from build123d import *

# Parameters (mm, degrees)
PAD_DEPTH            = 14
SKETCH001_R          = 12.7
POCKET_DEPTH         = 10
SKETCH002_R          = 3.2
POCKET001_DEPTH      = 20.001
POCKET001_DEPTH_BACK = -20.001
CHAMFER_SIZE         = 0.6


with BuildPart() as part:
    # Sketch → Pad (new body)
    with BuildSketch(Plane.XY):
        with BuildLine():
            Line((-36.717816, 3.612355), (-4.294539, 19.030888))
            ThreePointArc((4.294539, 19.030888), (0, 20), (-4.294539, 19.030888))
            Line((4.294539, 19.030888), (36.717816, 3.612355))
            ThreePointArc((36.717816, -3.612355), (39, 0), (36.717816, 3.612355))
            Line((36.717816, -3.612355), (4.294539, -19.030888))
            ThreePointArc((-4.294539, -19.030888), (0, -20), (4.294539, -19.030888))
            Line((-4.294539, -19.030888), (-36.717816, -3.612355))
            ThreePointArc((-36.717816, 3.612355), (-39, 0), (-36.717816, -3.612355))
        make_face()
    extrude(amount=PAD_DEPTH)

    # Sketch001 → Pocket (cut)
    with BuildSketch(Plane.XY):
        Circle(SKETCH001_R)
    extrude(amount=POCKET_DEPTH, mode=Mode.SUBTRACT)

    # Sketch002 → Pocket001 (cut, two sides)
    with BuildSketch(Plane(origin=(0, 0, -1), x_dir=(1, 0, 0), z_dir=(0, -1, 0))) as pocket001_sk:
        with Locations((0, 7)):
            Circle(SKETCH002_R)
    extrude(amount=-POCKET001_DEPTH, mode=Mode.SUBTRACT)
    extrude(pocket001_sk.sketch, amount=-POCKET001_DEPTH_BACK, mode=Mode.SUBTRACT)

    # Chamfer
    chamfer_edges = [part.edges().sort_by_distance(p)[0] for p in [
        (-20.506178, 11.321621, 0),
        (-39, 0, 0),
        (0, 20, 0),
        (-20.506178, -11.321621, 0),
        (20.506178, 11.321621, 0),
        (0, -20, 0),
        (39, 0, 0),
        (20.506178, -11.321621, 0),
        (-12.7, 0, 0),
        (-20.506178, 11.321621, 14),
        (0, 20, 14),
        (20.506178, 11.321621, 14),
        (39, 0, 14),
        (20.506178, -11.321621, 14),
        (0, -20, 14),
        (-20.506178, -11.321621, 14),
        (-39, 0, 14),
        (-3.2, -19.474175, 6),
        (-3.2, 19.474175, 6),
    ]]
    chamfer(chamfer_edges, length=CHAMFER_SIZE)


solid = part.part
Design review of the part built by this model. Coordinates are the model's own, in mm. A direction names the side the tool comes from. Coordinates: 2 decimals unless noted, no trailing zeros. Order: outer loops, then holes, each group sorted by start corner. A loop starts at its lowest first (then second) coordinate and runs counter-clockwise, first axis right, second up.
Item 1: Take a section at D-D, the plane x = 0. Count the separate pieces of the cut face and the enclosed holes in it, then the cut area to 3 significant figures.
Item 2: For faces 1 (the flat face through (0, 0, 10)), 2 (the cylindrical face through (39, 0, 7)), list the 3-axis set-ups (+Z, -Z, +X, -X, +Y, -Y) from which the entire face can be reached by the end or side of a thin tool; tool diameter is ignored.
Item 3: Take a section at A-A, the plane y = 0. Write out the cut boundary in (x, z).
Item 4: For pin 1 Ø8 at (x, z) = (-3.5, 10) entering from +Y; pin 2 Ø5 at (y, z) = (-11, 5) entering from -X; pin 3 Ø4 at (x, z) = (11.5, 6) entering from -Y; pin 4 Ø5 at (x, z) = (-2.5, 7) entering from -Y, all flat-tipped, find the tip position at first contact; note any pin that passes through.
Item 5: Take a section at C-C, the plane x = 32. Write out the cut boundary in (y, z), then the cut area to 3 significant figures.
Item 6: The part is to be moulded in two halves that separate along Z. For faces 3 (the cylindrical face through (-3.2, -15.8, 6.1)), 4 (the conical face through (-38.6, -0.1, 0.2)), 5 (the cylindrical face through (-3.2, 15.8, 6.1)), 6 (the flat face through (20.603, -10.939, 13.704)), say which applies: pulls with the +Z half, pulls with the -Z half, needs draft (parallel to the pull), parting line crosses it, or undercut.
Item 7: Take a section at B-B, the plane y = 15.5. Write out the cut boundary in (x, z).
Item 8: For line 1 (Z direction, x = 0, y = -16); line 2 (Z direction, x = -2.5, y = -16.5); line 3 (X direction, y = -15, z = 8.5), list the stretches that pass through material, from the lowest coordinate up.
The answers:
1. separate pieces: 3
1. enclosed holes: 0
1. area: 211 mm2
2. face 1: -Z
2. face 2: +Z, -Z, +X
3. outline: (-39, 0.6) - (-38.4, 0) - (-13.3, 0) - (-12.7, 0.6) - (-12.7, 10) - (12.7, 10) - (12.7, 0.6) - (13.3, 0) - (38.4, 0) - (39, 0.6) - (39, 13.4) - (38.4, 14) - (-38.4, 14) - (-39, 13.4) - close
4. pin 1: stops at y = 20
4. pin 2: stops at x = -26.44
4. pin 3: stops at y = -16.56
4. pin 4: stops at y = -19.85
5. outline: (-5.86, 0.6) - (-5.19, 0) - (5.19, 0) - (5.86, 0.6) - (5.86, 13.4) - (5.19, 14) - (-5.19, 14) - (-5.86, 13.4) - close
5. area: 163 mm2
6. face 3: undercut
6. face 4: pulls with the -Z half
6. face 5: undercut
6. face 6: pulls with the +Z half
7. outline: (-11.72, 0.6) - (-10.32, 0) - (10.32, 0) - (11.72, 0.6) - (11.72, 13.4) - (10.32, 14) - (-10.32, 14) - (-11.72, 13.4) - close; hole circle Ø6.4 at (0, 6)
8. line 1: z = 0 to 2.8, 9.2 to 14
8. line 2: z = 0 to 4, 8 to 14
8. line 3: x = -12.77 to -2, 2 to 12.77
